The listing builds one solid part. Answer for the finished solid, in the listing's coordinates (mm). Face numbers are marked on the shaded views. A direction names the side the tool comes from. Give positions to 0.01 mm unless a question says otherwise; leave off trailing zeros. Order: outer loops, then holes, each group sorted by start corner. A loop starts at its lowest first (then second) coordinate and runs counter-clockwise, first axis right, second up. Notation, with made-up numbers: (83, 11.25) - (94, 11.25) arc R18 cw to (94, 44.25) - close; hole circle Ø5 at (84.25, 5). An arc over 180 degrees is marked (long way). Answer in a Markdown table with one row per item.
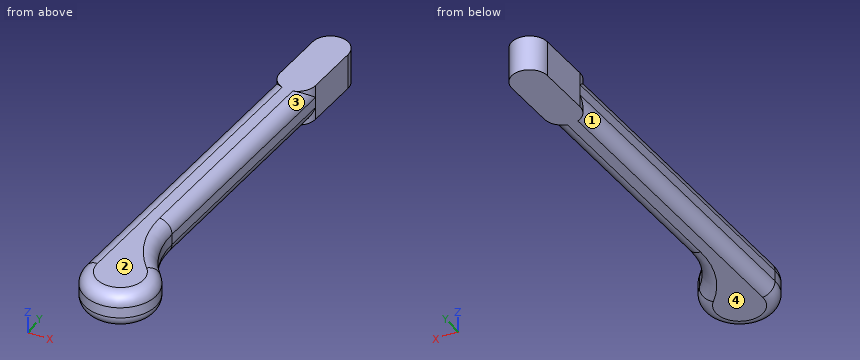
from build123d import *

# Parameters (mm, degrees)
EXTRUDE_1_DEPTH = 20
FILLET_1_R      = 7
EXTRUDE_2_DEPTH = 20


with BuildPart() as part:
    # 草图1 → 凸台-拉伸1 (new body)
    with BuildSketch(Plane.XY):
        with BuildLine():
            Line((-9.984555975, 0.555555556), (-19.969111951, -178.888888889))
            ThreePointArc((-19.969111951, -178.888888889), (6.717955109, -198.837969083), (14.759919727, -166.503897983))
            ThreePointArc((14.759919727, -166.503897983), (5.273090806, -150.735790608), (2.641695759, -132.52291348))
            Line((2.641695759, -132.52291348), (9.984555975, -0.555555556))
            ThreePointArc((9.984555975, -0.555555556), (0.555555556, 9.984555975), (-9.984555975, 0.555555556))
        make_face()
    extrude(amount=EXTRUDE_1_DEPTH)

    # 圆角1
    fillet_1_edges = [part.edges().sort_by_distance(p)[0] for p in [
        (6.313125867, -66.539234518, 20),
        (0.555555556, 9.984555975, 20),
        (-14.976833963, -89.166666667, 20),
        (6.717955109, -198.837969083, 20),
        (-14.976833963, -89.166666667, 0),
        (0.555555556, 9.984555975, 0),
        (6.313125867, -66.539234518, 0),
        (5.273090806, -150.735790608, 0),
        (6.717955109, -198.837969083, 0),
        (5.273090806, -150.735790608, 20),
    ]]
    fillet(fillet_1_edges, radius=FILLET_1_R)

    # 草图2 → 凸台-拉伸2 (add)
    with BuildSketch(Plane.XY):
        with BuildLine():
            Line((-9.984555975, 0.555555556), (-8.317889309, 30.509223482))
            ThreePointArc((-8.317889309, 30.509223482), (2.222222222, 39.938223901), (11.651222642, 29.39811237))
            Line((11.651222642, 29.39811237), (9.984555975, -0.555555556))
            ThreePointArc((9.984555975, -0.555555556), (-0.555555556, -9.984555975), (-9.984555975, 0.555555556))
        make_face()
    extrude(amount=EXTRUDE_2_DEPTH)


solid = part.part
Item 1: Each of these flat-tipped pins is pushed along its axis until it touches: P1, Ø10, axis at x = -6.5, y = -57, coming from the -Z side; P2, Ø1.5, axis at y = -141.5, z = 15, coming from the +X side; P3, Ø5, axis at x = -3, z = 8.5, coming from the +Y side; P4, Ø3, axis at y = -9, z = 16.5, coming from the +X side. Where does it stop, or does it pass through?
Answer block:
| item | result |
|---|---|
| P1 | z = 0 |
| P2 | x = 2.93 |
| P3 | y = 39.72 |
| P4 | x = 9.23 |
Item 2: Consider line 1 (Z direction, x = -15, y = -115); line 2 (X direction, y = -137.5, z = 11.75); line 3 (Z direction, x = -7.5, y = -63.5). Determine where each line is inside the solid, lowest interval first.
Answer block:
| item | result |
|---|---|
| line 1 | 2.78 to 17.22 |
| line 2 | -17.67 to 2.63 |
| line 3 | 0.07 to 19.93 |
Item 3: Which of the six approach directions +Z, -Z, +X, -X, +Y, -Y give full straight-line access (tool end or side, diameter ignored) to the marked faces 1 and 2?
Answer block:
| item | result |
|---|---|
| face 1 | -Z, -X |
| face 2 | +Z, +X, -X, +Y, -Y |
Item 4: Determine the mould class of the marked faces 3 and 4 for opening direction Y: pulls with the +Y half, pulls with the -Y half, needs draft (parallel to the pull), parting line crosses it, or undercut.
Answer block:
| item | result |
|---|---|
| face 3 | undercut |
| face 4 | needs draft |
Item 5: Find section A-A on z = 10.25. Write down the section's boundary in (x, y).
Answer block:
| item | result |
|---|---|
| outline | (-19.97, -178.89) arc R20 ccw (long way) to (14.76, -166.5) arc R46.53 cw to (2.64, -132.52) - (11.65, 29.4) arc R10 ccw to (-8.32, 30.51) - close |
